CAD build for the part. Positions are in the model's coordinates, mm. Round coordinates to 2 decimals unless told otherwise and drop trailing zeros. Loops run counter-clockwise (first coordinate to the right, second up) from the corner with the lowest first, then second, coordinate; pieces in that order, holes last.
from build123d import *

# Parameters (mm, degrees)
SKETCH3_R               = 3.175
BOSS_EXTRUDE1_DEPTH     = 304.8
CHAMFER1_SIZE           = 0.635
CUT_EXTRUDE1_START      = -118.919625
SKETCH4_R               = 3.175
CUT_EXTRUDE1_DEPTH      = 491.680375
SKETCH5_R               = 0.5953125
CUT_EXTRUDE2_DEPTH      = 4.175
CUT_EXTRUDE2_DEPTH_BACK = 4.175


with BuildPart() as part:
    # Sketch3 → Boss-Extrude1 (new body, symmetric)
    with BuildSketch(Plane.XY):
        Circle(SKETCH3_R)
    extrude(amount=BOSS_EXTRUDE1_DEPTH, both=True)

    # Chamfer1
    chamfer1_edges = [part.edges().sort_by_distance(p)[0] for p in [
        (-3.175, 0, -304.8),
        (-3.175, 0, 304.8),
    ]]
    chamfer(chamfer1_edges, length=CHAMFER1_SIZE)

    # Sketch4 → Cut-Extrude1 (cut, through all)
    with BuildSketch(Plane.XY.offset(304.8).offset(CUT_EXTRUDE1_START)):
        Circle(SKETCH4_R)
    extrude(amount=-CUT_EXTRUDE1_DEPTH, mode=Mode.SUBTRACT)

    # Sketch5 → Cut-Extrude2 (cut, two sides)
    with BuildSketch(Plane(origin=(0, 0, 0), x_dir=(1, 0, 0), z_dir=(0, 1, 0))) as cut_extrude2_sk:
        with Locations((0, -187.467875)):
            Circle(SKETCH5_R)
        with Locations((0, -303.2125)):
            Circle(SKETCH5_R)
    extrude(amount=CUT_EXTRUDE2_DEPTH, mode=Mode.SUBTRACT)
    extrude(cut_extrude2_sk.sketch, amount=-CUT_EXTRUDE2_DEPTH_BACK, mode=Mode.SUBTRACT)


solid = part.part
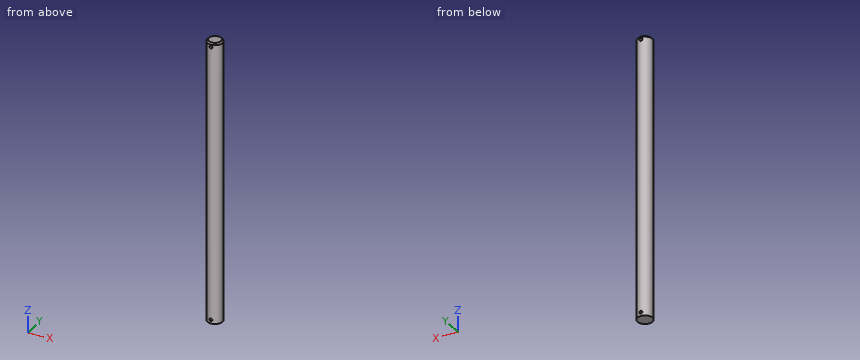
Item 1: Flat gauge pins, fed straight in: P1, Ø1.5, axis at y = 2, z = 214, coming from the -X side; P2, Ø2, axis at x = 2, z = 204.5, coming from the +Y side. Where does each tip first touch, or does it go through?
Verdict:
P1: stops at x = -2.92
P2: stops at y = 3.01
Item 2: Wall check: L1, parallel to Z at x = 0, y = -1.95; L2, parallel to Z at x = 0.5, y = 1; L3, parallel to X at y = 0.25, z = 263.5. Give the ranges that are in metal, low to high.
Verdict:
L1: z = 185.88 to 186.87, 188.06 to 302.62, 303.81 to 304.8
L2: z = 185.88 to 187.14, 187.79 to 302.89, 303.54 to 304.8
L3: x = -3.17 to 3.17
Item 3: Cut at B-B (y = 1). State how many separate pieces and enclosed holes the cut face has, plus the area to 3 significant figures.
Verdict:
separate pieces: 1
enclosed holes: 2
area: 714 mm2
Item 4: Cut at A-A (z = 247.5). List the corners of the cut face in (x, y) (3 decimals), plus the area to 3 significant figures.
Verdict:
outline: circle Ø6.35 at (0, 0)
area: 31.7 mm2
